Check sheet for the modelled part. Datum: model origin and axes. Units: mm. Face numbers are marked on the shaded views. Round coordinates to 2 decimals unless told otherwise and drop trailing zeros. Loops run counter-clockwise (first coordinate to the right, second up) from the corner with the lowest first, then second, coordinate; pieces in that order, holes last. Notation, with made-up numbers: (57, 39) - (83, 39) arc R25 ccw to (83, 72) - close; hole circle Ø5 at (34.5, -16.5). An arc over 180 degrees is marked (long way). Put each result on its own line as item: value. Start each with the question number.
Item 1: Draft check along Z on the marked faces 1, 2 and 3. Enter one of: pulls with the +Z half, pulls with the -Z half, needs draft (parallel to the pull), parting line crosses it, or undercut.
Item 2: Material ranges on line 1 along Y through (x, z) = (4.5, -25.5); line 2 along Z through (x, y) = (0, -1); line 3 along X through (y, z) = (21, -24.5), recorded low to high.
Item 3: Section check C-C, the plane z = 16. Give the number of separate pieces and of enclosed holes in the cut face, and give its area (3 significant figures).
Item 4: Section check B-B, the plane y = 22. Record the cut outline in (x, z).
Item 5: Section check A-A, the plane x = -8. Record the cut outline in (y, z).
Item 6: Gauge pin test, flat ends, axial feed: pin 1 Ø10 at (x, z) = (4, -17) entering from +Y; pin 2 Ø12 at (x, z) = (-10.5, -13) entering from +Y. Record the tip position at first contact, or that the pin passes through.
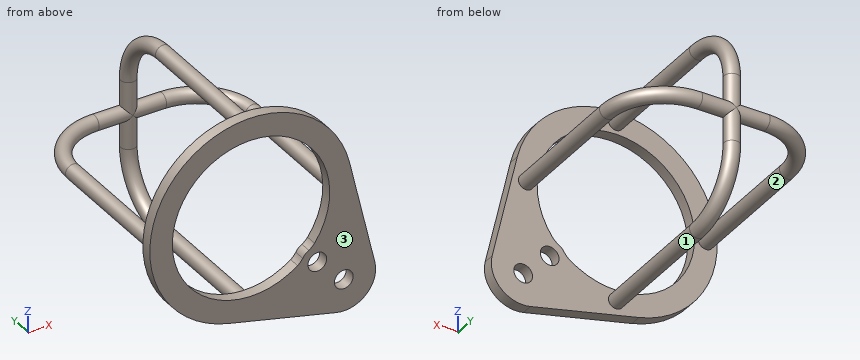
from build123d import *

# Parameters (mm, degrees)
ESQUISSE2_R                  = 2
R_P_TITION_CIRCULAIRE1_COUNT = 4
ESQUISSE4_R                  = 2.5
BOSS_EXTRU_1_DEPTH           = 3
CONG_1_R                     = 5


with BuildPart() as part:
    # Balayage1: sweep along a path in Esquisse1
    with BuildLine(Plane.XY) as balayage1_path:
        Line((0, 50), (9, 50))
        ThreePointArc((9, 50), (19.606601718, 45.606601718), (24, 35))
        Line((24, 35), (24, 0))
    # Esquisse2 → Balayage1 (sweep)
    with BuildSketch(Plane(origin=(0, 0, 0), x_dir=(1, 0, 0), z_dir=(0, 1, 0))):
        with Locations((24, 0)):
            Circle(ESQUISSE2_R)
    balayage1 = sweep(path=balayage1_path.line)

    # Répétition circulaire1: Balayage1 ×4 about axis
    r_p_tition_circulaire1_axis = Axis((0, 0, 0), (0, 1, 0))
    for i in range(1, R_P_TITION_CIRCULAIRE1_COUNT):
        add(balayage1.rotate(r_p_tition_circulaire1_axis, i * 360 / R_P_TITION_CIRCULAIRE1_COUNT))

    # Esquisse4 → Boss.-Extru.1 (add)
    with BuildSketch(Plane.XZ):
        with BuildLine():
            Line((26.298310212, 6.115462371), (33.027835001, -22.823499188))
            ThreePointArc((33.027835001, -22.823499188), (30.759144982, -30.759144982), (22.823499188, -33.027835001))
            Line((22.823499188, -33.027835001), (-6.115462371, -26.298310212))
            ThreePointArc((-6.115462371, -26.298310212), (-19.091883092, 19.091883092), (26.298310212, 6.115462371))
        make_face()
        with Locations((17.67766953, -17.67766953)):
            Circle(ESQUISSE4_R, mode=Mode.SUBTRACT)
        with Locations((24.748737342, -24.748737342)):
            Circle(ESQUISSE4_R, mode=Mode.SUBTRACT)
        with BuildLine():
            ThreePointArc((13.454452036, -16.123824621), (14.495689014, -14.495689014), (16.123824621, -13.454452036))
            ThreePointArc((16.123824621, -13.454452036), (-14.849242405, 14.849242405), (13.454452036, -16.123824621))
        make_face(mode=Mode.SUBTRACT)
    extrude(amount=BOSS_EXTRU_1_DEPTH)

    # Congé1
    cong_1_edges = [part.edges().sort_by_distance(p)[0] for p in [
        (13.454452036, -1.5, -16.123824621),
        (16.123824621, -1.5, -13.454452036),
    ]]
    fillet(cong_1_edges, radius=CONG_1_R)


solid = part.part
Check result:
1. face 1: undercut
1. face 2: parting line crosses it
1. face 3: needs draft
2. line 1: -3 to 0
2. line 2: -27.72 to -21, 21 to 27
2. line 3: -1.94 to 1.94
3. separate pieces: 3
3. enclosed holes: 0
3. area: 63.1 mm²
4. outline: circle Ø4 at (-24, 0); circle Ø4 at (0, -24); circle Ø4 at (0, 24); circle Ø4 at (24, 0)
5. outline: (-3, -25.79) - (0, -25.79) - (0, -19.42) - (-3, -19.42) - close; (-3, 19.42) - (0, 19.42) - (0, 25.79) - (-3, 25.79) - close; circle Ø4 at (50, 0)
6. pin 1: y = 51.35
6. pin 2: y = 0
